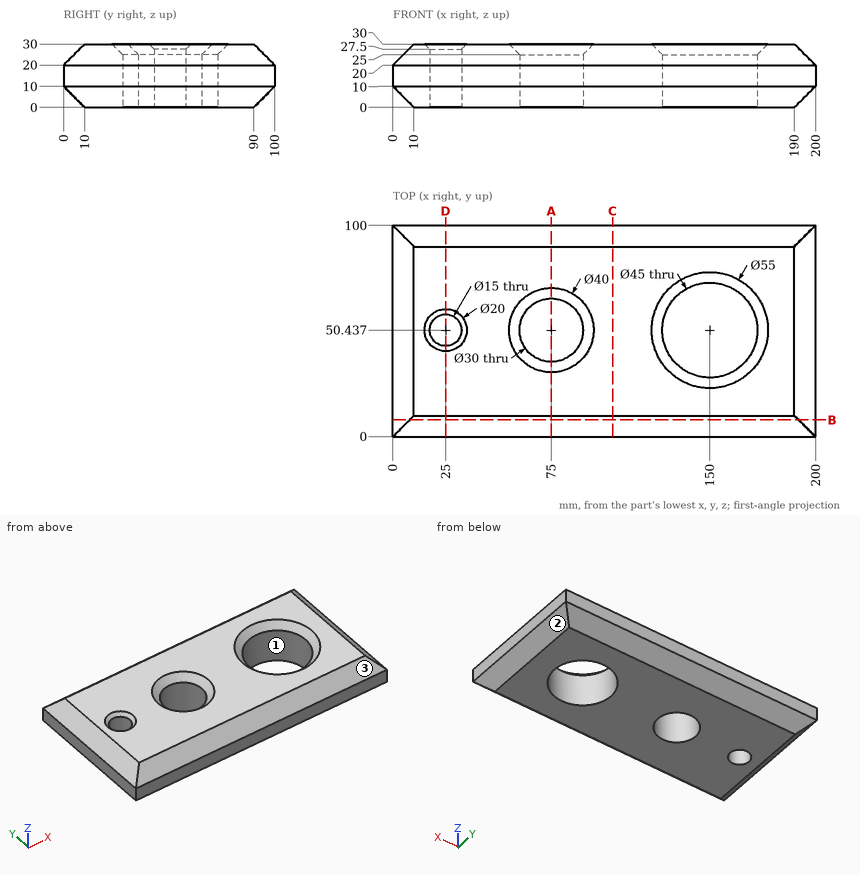
Job drawing, mm, ordinate dimensions from the low corner. One solid piece. Give positions to 0.01 mm unless a question says otherwise; leave off trailing zeros. Write each loop counter-clockwise with the first axis right and the second up, starting at its lowest first coordinate (ties: lowest second). Pieces come first, ordered by that corner, then holes. Notation, with made-up numbers: (0.25, 69.25) - (36.25, 69.25) arc R24 ccw to (36.25, 106.25) - close; hole circle Ø11 at (-5.5, 27). An arc over 180 degrees is marked (long way). Answer as CSV lines item,"result".
1. Band-saw the part on B-B (y = 8). Write the cut outline in (x, z).
Responses:
outline,"(0, 10) - (8, 2) - (192, 2) - (200, 10) - (200, 20) - (192, 28) - (8, 28) - (0, 20) - close"
2. Band-saw the part on A-A (x = 75). Write the cut outline in (y, z), and give its area (4 significant figures).
Responses:
outline,"(0, 10) - (10, 0) - (35.44, 0) - (35.44, 25) - (30.44, 30) - (10, 30) - (0, 20) - close; (65.44, 0) - (90, 0) - (100, 10) - (100, 20) - (90, 30) - (70.44, 30) - (65.44, 25) - close"
area,"1,875 mm2"
3. Band-saw the part on D-D (x = 25). Write the cut outline in (y, z).
Responses:
outline,"(0, 10) - (10, 0) - (42.94, 0) - (42.94, 27.5) - (40.44, 30) - (10, 30) - (0, 20) - close; (57.94, 0) - (90, 0) - (100, 10) - (100, 20) - (90, 30) - (60.44, 30) - (57.94, 27.5) - close"
4. Two-plate mould, pull along X, no slides. Class the marked faces 1, 2 and 3: +X half, -X half, draft (parallel to the pull), parting line (faces both ways), or undercut.
Responses:
face 1,"undercut"
face 2,"+X half"
face 3,"draft"
5. Pin check, flat tips, straight feed: pin 1 (12 mm diameter, centred on x = 100, y = 86, fed in from -Z); pin 2 (3 mm diameter, centred on y = 73.5, z = 24.5, fed in from -X); pin 3 (4 mm diameter, centred on y = 19, z = 25.5, fed in from +X); pin 4 (1.5 mm diameter, centred on x = 132, y = 31, fed in from +Z). Stop position of each tip, or through.
Responses:
pin 1,"stops at z = 0"
pin 2,"stops at x = 3"
pin 3,"stops at x = 196.5"
pin 4,"stops at z = 29.74"
6. Band-saw the part on C-C (x = 104). Write the cut outline in (y, z), and give its area (3 significant figures).
Responses:
outline,"(0, 10) - (10, 0) - (90, 0) - (100, 10) - (100, 20) - (90, 30) - (10, 30) - (0, 20) - close"
area,"2,800 mm2"
7. Drill centre lines: L1, parallel to Y at x = 150, z = 18.5; L2, parallel to Y at x = 75.5, z = 19.75 (1 decimal); L3, parallel to X at y = 46, z = 18 (1 decimal). Where is each one in solid material? Low to high. Write a range as [from, to].
Responses:
L1,"y = [0, 27.94], [72.94, 100]"
L2,"y = [0, 35.4], [65.4, 100]"
L3,"x = [0, 19], [31, 60.7], [89.3, 127.9], [172.1, 200]"
